Can you work these out from the model? Positions are in its coordinate system, mm. Round coordinates to 2 decimals unless told otherwise and drop trailing zeros. Order: outer loops, then holes, each group sorted by start corner. A loop starts at its lowest first (then second) coordinate and runs counter-clockwise, first axis right, second up. Notation, with made-up numbers: M 76,-35 L 106,-35 A22 ccw 106,-22 Z; hole C 73,18.25 d3. An arc over 180 degrees is marked long. Answer as a JSON object with one key per item and string values. Group by question number.
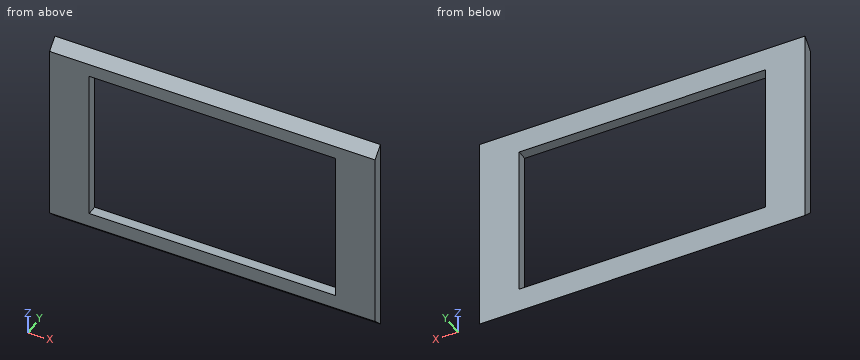
```python
from build123d import *

# Parameters (mm, degrees)
SKETCH1_W           = 100
SKETCH1_H           = 5
BOSS_EXTRUDE1_DEPTH = 300
CUT_EXTRUDE1_DEPTH  = 300
SKETCH3_W           = 121
SKETCH3_H           = 76.5
CUT_EXTRUDE2_DEPTH  = 5
CUT_EXTRUDE3_DEPTH  = 300
SKETCH5_W           = 70
SKETCH5_H           = 100
CUT_EXTRUDE4_DEPTH  = 5


with BuildPart() as part:
    # Sketch1 → Boss-Extrude1 (new body)
    with BuildSketch(Plane(origin=(0, 0, 0), x_dir=(0, 0, -1), z_dir=(1, 0, 0))):
        Rectangle(SKETCH1_W, SKETCH1_H)
    extrude(amount=BOSS_EXTRUDE1_DEPTH)

    # Sketch2 → Cut-Extrude1 (cut)
    with BuildSketch(Plane(origin=(300, 0, 0), x_dir=(0, 0, -1), z_dir=(1, 0, 0))):
        Polygon((-50, 2.5), (-45, -2.5), (-50, -2.5), align=None)
    extrude(amount=-CUT_EXTRUDE1_DEPTH, mode=Mode.SUBTRACT)

    # Sketch3 → Cut-Extrude2 (cut)
    with BuildSketch(Plane(origin=(0, 2.5, 0), x_dir=(1, 0, 0), z_dir=(0, 1, 0))):
        with Locations((150, -0.25)):
            Rectangle(SKETCH3_W, SKETCH3_H)
    extrude(amount=-CUT_EXTRUDE2_DEPTH, mode=Mode.SUBTRACT)

    # Sketch4 → Cut-Extrude3 (cut)
    with BuildSketch(Plane(origin=(300, 0, 0), x_dir=(0, 0, -1), z_dir=(1, 0, 0))):
        Polygon((50, 2.5), (45, -2.5), (50, -2.5), align=None)
    extrude(amount=-CUT_EXTRUDE3_DEPTH, mode=Mode.SUBTRACT)

    # Sketch5 → Cut-Extrude4 (cut)
    with BuildSketch(Plane(origin=(0, 2.5, 0), x_dir=(1, 0, 0), z_dir=(0, 1, 0))):
        with Locations((35, 0)):
            Rectangle(SKETCH5_W, SKETCH5_H)
        with Locations((265, 0)):
            Rectangle(SKETCH5_W, SKETCH5_H)
    extrude(amount=-CUT_EXTRUDE4_DEPTH, mode=Mode.SUBTRACT)


solid = part.part
```
1) I need wall thicknesses on line 1 along X through (y, z) = (-0.2, -4.5); line 2 along Z through (x, y) = (195.5, 0.85); line 3 along Z through (x, y) = (125.5, 2.1). Which ranges of each line are inside material? Lowest first, please.
2) If we section it at B-B on y = 0.45: Write out the boundary of the cut face in (x, z).
3) If we section it at A-A on z = -14: Write out the boundary of the cut face in (x, y).
4) If we section it at C-C on x = 168.5: Write out the boundary of the cut face in (y, z), plus the area to 3 significant figures.
5) For pin 1 (2.5 mm diameter, centred on x = 167, y = 1, fed in from -Z); pin 2 (1.5 mm diameter, centred on x = 147, y = 1, fed in from +Z), each with a flat end and sliding along its axis, tell me the tip position at first contact or that it passes through.
Findings:
{
 "1": {"line 1": "x = 70 to 89.5, 210.5 to 230", "line 2": "z = -48.35 to -38, 38.5 to 48.35", "line 3": "z = -49.6 to -38, 38.5 to 49.6"},
 "2": {"outline": "M 70,-47.95 L 230,-47.95 L 230,47.95 L 70,47.95 Z; hole M 89.5,-38 L 210.5,-38 L 210.5,38.5 L 89.5,38.5 Z"},
 "3": {"outline": "M 70,-2.5 L 89.5,-2.5 L 89.5,2.5 L 70,2.5 Z; M 210.5,-2.5 L 230,-2.5 L 230,2.5 L 210.5,2.5 Z"},
 "4": {"outline": "M -2.5,-45 L 2.5,-50 L 2.5,-38 L -2.5,-38 Z; M -2.5,38.5 L 2.5,38.5 L 2.5,50 L -2.5,45 Z", "area": "92.5 mm^2"},
 "5": {"pin 1": "stops at z = -49.75", "pin 2": "stops at z = 49.25"}
}
